The listing builds one solid part. Answer for the finished solid, in the listing's coordinates (mm). A direction names the side the tool comes from. Round coordinates to 2 decimals unless told otherwise and drop trailing zeros. Write each loop counter-clockwise with the first axis right and the second up, starting at its lowest first coordinate (ties: lowest second). Pieces come first, ordered by that corner, then holes. Notation, with made-up numbers: M 29,88 L 83,88 A18 cw 83,97 Z; hole C 36,-7.5 d9. An arc over 180 degrees is marked long. Write each question's results on one line, items separated by ' | '.
from build123d import *

# Parameters (mm, degrees)
F0_W     = 140.2715
F0_H     = 14.3383389879
F0_H_2   = 14.224
F1_DEPTH = 68.326
F2_W     = 29.21
F2_H     = 14.3383389879
F3_DEPTH = 140.2725
F4_W     = 47.3744553204
F4_H     = 60.4247975121
F5_DEPTH = 140.2725
F8_DEPTH = 19.05


with BuildPart() as f1:
    # F0 (on Front) → F1 (new body)
    with BuildSketch(Plane.XZ):
        with Locations((-16.5940149384, -7.1691694939)):
            Rectangle(F0_W, F0_H)
        with Locations((-16.5940149384, 7.112)):
            Rectangle(F0_W, F0_H_2)
        with BuildLine():
            Line((-86.7297649384, 39.7636610121), (-86.7297649384, 14.224))
            Line((-86.7297649384, 14.224), (53.5417350616, 14.224))
            Line((53.5417350616, 14.224), (-50.5952610901, 62.7838788028))
            ThreePointArc((-50.5952610901, 62.7838788028), (-74.9771749904, 61.1858037358), (-86.7297649384, 39.7636610121))
        make_face()
    extrude(amount=F1_DEPTH)

    # F2 (on face) → F3 (cut, through all)
    with BuildSketch(Plane.YZ.offset(53.5417350616)):
        with Locations((-53.721, -7.1691694939)):
            Rectangle(F2_W, F2_H)
    extrude(amount=-F3_DEPTH, mode=Mode.SUBTRACT)

    # F4 (on face) → F5 (cut, through all)
    with BuildSketch(Plane.YZ.offset(53.5417350616)):
        with Locations((-71.9472276602, 44.436398756)):
            Rectangle(F4_W, F4_H)
    extrude(amount=-F5_DEPTH, mode=Mode.SUBTRACT)

    # F7 (on offset) → F8 (cut)
    with BuildSketch(Plane.XZ.offset(15.748)):
        Polygon((-29.5870655151, 23.7108610121), (-8.6876207146, 68.5298650214), (-100.3249382806, 74.6821943388), (-100.3249382806, 23.7108610121), align=None)
    extrude(amount=F8_DEPTH, mode=Mode.SUBTRACT)

    # F10 (on offset) → F11 (revolve, cut)
    with BuildSketch(Plane.XZ.offset(22.225)):
        Polygon((-5.9485983328, 10.5759030094), (11.6252099843, 48.2630565653), (0, 53.6839810086), (-14.3165883004, 22.9819583202), align=None)
    revolve(axis=Axis((2.8383058257, -22.225, 29.4194797873), (-0.4226182617, 0, -0.906307787)), mode=Mode.SUBTRACT)


solid = f1.part
1) Each of these flat-tipped pins is pushed along its axis until it touches: pin 1 (14.5 mm diameter, centred on x = -31.5, y = -52, fed in from -Z); pin 2 (15.5 mm diameter, centred on x = -3, z = 30, fed in from -Y); pin 3 (6 mm diameter, centred on x = -18, y = -57.5, fed in from +Z). Where does it stop, or does it pass through?
Return value:
pin 1: z = 0 | pin 2: y = -48.26 | pin 3: z = 14.22
2) Section D-D (x = 25) is taken. Determine the outline of the cut face in (y, z).
Return value:
outline: M -68.33,0 L -39.12,0 L -39.12,-14.34 L 0,-14.34 L 0,27.53 L -48.26,27.53 L -48.26,14.22 L -68.33,14.22 Z
3) Section A-A (z = 52) is taken. Determine the outline of the cut face in (x, y).
Return value:
outline: M -83.59,-48.26 L -27.47,-48.26 L -27.47,-34.8 L -83.59,-34.8 Z; M -83.59,-15.75 L -27.47,-15.75 L -27.47,0 L -83.59,0 Z
4) Section B-B (x = -25.5) is taken. Determine the outline of the cut face in (y, z).
Return value:
outline: M -68.33,0 L -39.12,0 L -39.12,-14.34 L 0,-14.34 L 0,51.08 L -15.75,51.08 L -15.75,32.48 L -34.8,32.48 L -34.8,51.08 L -48.26,51.08 L -48.26,14.22 L -68.33,14.22 Z
5) The mould has two halves that part along Y. Classify faces 6 (the face through (-16, -54, 0)), 7 (the face through (-18, -68.326, 7)), 8 (the face through (-59, -25, 23.711)): +Y half, -Y half, draft (parallel to the pull), parting line (faces both ways), or undercut.
Return value:
face 6: draft | face 7: -Y half | face 8: undercut
6) Section C-C (y = -6) is taken. Determine the outline of the cut face in (x, z), then the cut area to 3 significant figures.
Return value:
outline: M -86.73,-14.34 L 53.54,-14.34 L 53.54,14.22 L -50.6,62.78 A25.4 ccw -86.73,39.76 Z | area: 8,230 mm²
7) Find the intervals of material crossed by line 1 (Y direction, x = -44, z = 36); line 2 (Z direction, x = -64, y = -61.5); line 3 (Z direction, x = -40, y = -33.5), in increasing order.
Return value:
line 1: -48.26 to -34.8, -15.75 to 0 | line 2: 0 to 14.22 | line 3: -14.34 to 23.71
8) A tool of negligible diameter and unlimited length cuts with its end or side. For faces 1 (the face through (-6.285, -24.042, 12.091)), 2 (the face through (-53, -34.798, 40)), 3 (the face through (-16, -39.116, -7)), 4 (the face through (-31, -48.26, 34)), 5 (the face through (-74.67, -7.76, 61.38)), from which of +Z, -Z, +X, -X, +Y, -Y can it reach the whole face along a straight path? Write none if from no direction.
Return value:
face 1: none | face 2: +Z, -X | face 3: -Z, +X, -X, -Y | face 4: +Z, +X, -X, -Y | face 5: +Z, +Y, -Y
